The figure shows three views and two pictorial views of one solid part (mm, origin at its lowest corner). Answer the questions. A direction names the side the tool comes from. Round coordinates to 2 decimals unless told otherwise and drop trailing zeros. Order: outer loops, then holes, each group sorted by start corner. A loop starts at its lowest first (then second) coordinate and runs counter-clockwise, first axis right, second up. Notation, with made-up numbers: M 38,5 L 84,5 A27 cw 84,42 Z; hole C -34,-28.75 d10. An arc over 180 degrees is marked long. Return JSON: item names as keys, results as strings.
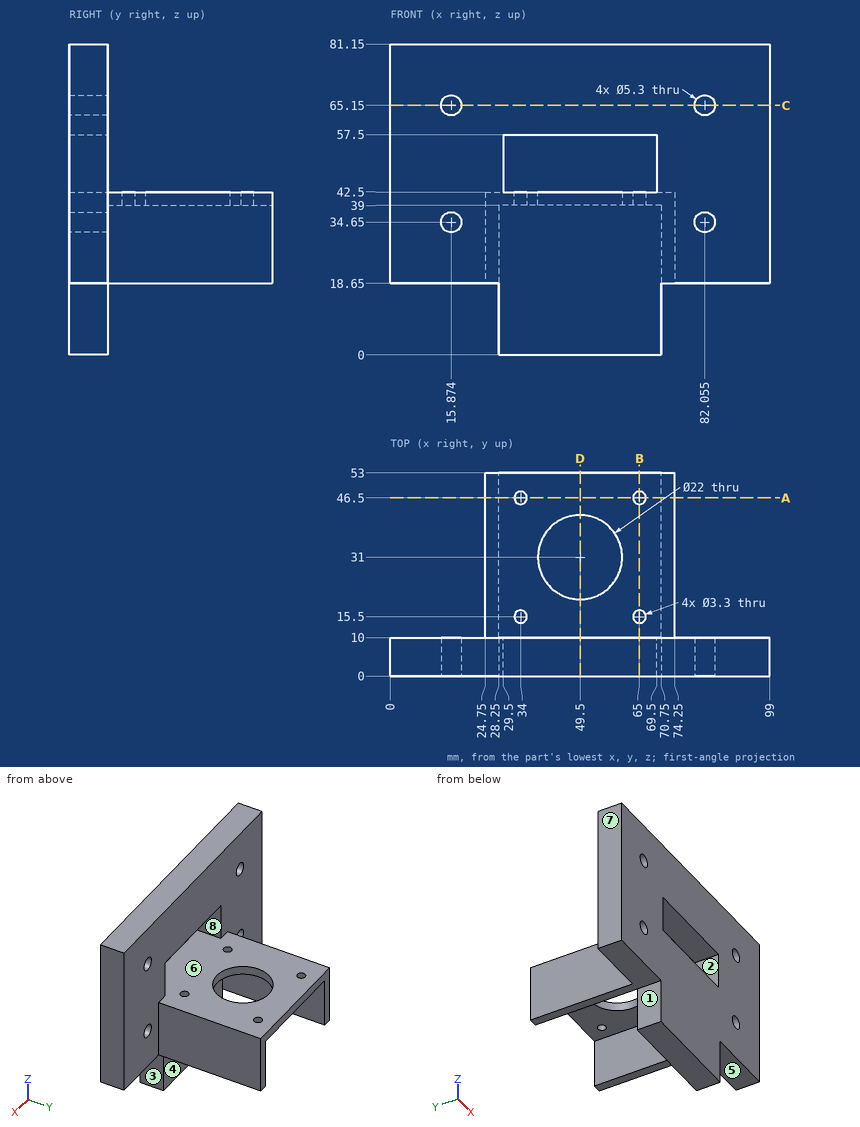
Item 1: Which of the six approach directions +Z, -Z, +X, -X, +Y, -Y give full straight-line access (tool end or side, diameter ignored) to the marked faces 1, 2, 3 and 4?
Output:
{"face 1": "-Z, -X, +Y, -Y", "face 2": "+Y, -Y", "face 3": "-Z, +X, +Y, -Y", "face 4": "-Z, +Y"}
Item 2: The mould has two halves that part along Z. Classify the marked faces 5, 6, 7 and 8: pulls with the +Z half, pulls with the -Z half, needs draft (parallel to the pull), parting line crosses it, or undercut.
Output:
{"face 5": "pulls with the -Z half", "face 6": "undercut", "face 7": "needs draft", "face 8": "undercut"}
Item 3: Consider line 1 along X through (y, z) = (43.5, 26); line 2 along X through (y, z) = (3, 65); line 3 along Y through (x, z) = (49.5, 40.95). Determine where each line is inside the solid, lowest interval first. Write a range as [from, to].
Output:
{"line 1": "x = [24.75, 28.25], [70.75, 74.25]", "line 2": "x = [0, 13.23], [18.52, 79.41], [84.7, 99]", "line 3": "y = [0, 20], [42, 53]"}
Item 4: Find section C-C (z = 65.15). Determine the outline of the cut face in (x, y) (1 decimal).
Output:
{"outline": "M 0,0 L 13.2,0 L 13.2,10 L 0,10 Z; M 18.5,0 L 79.4,0 L 79.4,10 L 18.5,10 Z; M 84.7,0 L 99,0 L 99,10 L 84.7,10 Z"}
Item 5: Each of these flat-tipped pins is pushed along its axis until it touches: pin 1 (13 mm diameter, centred on x = 59, y = 33.5, fed in from -Z); pin 2 (3 mm diameter, centred on y = 5.5, z = 11, fed in from -X); pin 3 (22.5 mm diameter, centred on x = 18, y = 15.5, fed in from -Z). Where does it stop, or does it pass through?
Output:
{"pin 1": "stops at z = 39", "pin 2": "stops at x = 28.25", "pin 3": "stops at z = 18.65"}
Item 6: Find section D-D (x = 49.5). Determine the outline of the cut face in (y, z).
Output:
{"outline": "M 0,0 L 10,0 L 10,39 L 20,39 L 20,42.5 L 0,42.5 Z; M 0,57.5 L 10,57.5 L 10,81.15 L 0,81.15 Z; M 42,39 L 53,39 L 53,42.5 L 42,42.5 Z"}
Item 7: Find section A-A (y = 46.5). Determine the outline of the cut face in (x, z).
Output:
{"outline": "M 24.75,18.65 L 28.25,18.65 L 28.25,39 L 32.35,39 L 32.35,42.5 L 24.75,42.5 Z; M 35.65,39 L 63.35,39 L 63.35,42.5 L 35.65,42.5 Z; M 66.65,39 L 70.75,39 L 70.75,18.65 L 74.25,18.65 L 74.25,42.5 L 66.65,42.5 Z"}
Item 8: Find section B-B (x = 65). Determine the outline of the cut face in (y, z), plus the area to 3 significant figures.
Output:
{"outline": "M 0,0 L 10,0 L 10,39 L 13.85,39 L 13.85,42.5 L 0,42.5 Z; M 0,57.5 L 10,57.5 L 10,81.15 L 0,81.15 Z; M 17.15,39 L 44.85,39 L 44.85,42.5 L 17.15,42.5 Z; M 48.15,39 L 53,39 L 53,42.5 L 48.15,42.5 Z", "area": "789 mm^2"}
